The listing builds one solid part. Answer for the finished solid, in the listing's coordinates (mm). A direction names the side the tool comes from. Round coordinates to 2 decimals unless told otherwise and drop trailing zeros. Write each loop counter-clockwise with the first axis right and the second up, starting at its lowest first coordinate (ties: lowest second). Pieces come first, ordered by that corner, then holes.
(1) A cutting plane is placed at B-B, the plane z = 0.75. Give the vertices of the cut face in (x, y).
(2) For faces 1 (the face through (-1.462, -0.035, 1.756)), 2 (the face through (-0.1, 2.5, 0.3)), determine the directions among +Z, -Z, +X, -X, +Y, -Y from which every point of the face is accessible in a straight line to the end or side of a thin tool.
(3) A cutting plane is placed at C-C, the plane x = -1.25. Give the vertices of the cut face in (y, z), and give its area (3 significant figures).
(4) A cutting plane is placed at D-D, the plane z = 0.15. Give the vertices of the cut face in (x, y).
(5) The mould has two halves that part along X. Classify faces 3 (the face through (7, 0, 0.5)), 4 (the face through (-5, 0, 2)), 5 (the face through (1.438, -0.035, 1.742)): +X half, -X half, draft (parallel to the pull), parting line (faces both ways), or undercut.
(6) A cutting plane is placed at A-A, the plane y = 0.9. Give the vertices of the cut face in (x, z), and give its area (3 significant figures).
(7) Find the intervals of material crossed by probe 1 along X at (y, z) = (1.15, 0.75); probe 2 along X at (y, z) = (1.7, 0.9); probe 3 along Z at (x, y) = (-0.75, 1.3), in increasing order.
from build123d import *

# Parameters (mm, degrees)
F0_W     = 15
F0_H     = 5
F1_DEPTH = 2
F2_W     = 4.732864
F2_H     = 0.538756
F3_DEPTH = 5.001
F4_SIZE  = 1


with BuildPart() as f1:
    # F0 (on Top) → F1 (new body)
    with BuildSketch(Plane.XY):
        Rectangle(F0_W, F0_H)
    extrude(amount=F1_DEPTH)

    # F2 (on face) → F3 (cut, through all)
    with BuildSketch(Plane.XZ.offset(2.5)):
        with BuildLine():
            ThreePointArc((-2.366432, 2), (-1.449917, 1.749193), (-0.788811, 1.066667))
            ThreePointArc((-0.788811, 1.066667), (0, 0.6), (0.788811, 1.066667))
            ThreePointArc((0.788811, 1.066667), (1.449917, 1.749193), (2.366432, 2))
            Line((2.366432, 2), (-2.366432, 2))
        make_face()
        with Locations((0, 2.269378)):
            Rectangle(F2_W, F2_H)
    extrude(amount=-F3_DEPTH, mode=Mode.SUBTRACT)

    # F4
    f4_edges = [f1.edges().sort_by_distance(p)[0] for p in [
        (-7.5, 0, 0),
        (7.5, 0, 0),
    ]]
    chamfer(f4_edges, length=F4_SIZE)


solid = f1.part
Solutions:
1. outline: (-7.25, -2.5) - (-0.5, -2.5) - (-0.5, 2.5) - (-7.25, 2.5) - close; (0.5, -2.5) - (7.25, -2.5) - (7.25, 2.5) - (0.5, 2.5) - close
2. face 1: +Z, +Y, -Y
2. face 2: +Z, -Z, +X, -X, +Y
3. outline: (-2.5, 0) - (2.5, 0) - (2.5, 1.61) - (-2.5, 1.61) - close
3. area: 8.06 mm2
4. outline: (-6.65, -2.5) - (6.65, -2.5) - (6.65, 2.5) - (-6.65, 2.5) - close
5. face 3: +X half
5. face 4: draft
5. face 5: undercut
6. outline: (-7.5, 1) - (-6.5, 0) - (6.5, 0) - (7.5, 1) - (7.5, 2) - (2.37, 2) arc R1.8 ccw to (0.79, 1.07) arc R0.9 cw to (-0.79, 1.07) arc R1.8 ccw to (-2.37, 2) - (-7.5, 2) - close
6. area: 26.2 mm2
7. probe 1: x = -7.25 to -0.5, 0.5 to 7.25
7. probe 2: x = -7.4 to -0.67, 0.67 to 7.4
7. probe 3: z = 0 to 1
